Read the model definition and answer for the solid it produces. Units are mm, in the model's axes. A direction names the side the tool comes from. Give positions to 0.01 mm unless a question says otherwise; leave off trailing zeros. Loops run counter-clockwise (first coordinate to the right, second up) from the corner with the lowest first, then second, coordinate; pieces in that order, holes last.
(1) Find section C-C, the plane z = -3.25. Write down the section's boundary in (x, y), then the cut area to 3 significant figures.
(2) Each of these flat-tipped pins is pushed along its axis until it touches: P1, Ø2.5, axis at x = -12, y = 3, coming from the -Z side; P2, Ø1, axis at y = 0.5, z = 1, coming from the +X side; P3, Ø2, axis at x = -3, y = 3, coming from the -Z side. Where does it stop, or does it pass through?
(3) Straight lines are drawn through the part: probe 1 along X at (y, z) = (1.5, -1); probe 2 along X at (y, z) = (3.6, 3.75); probe 3 along Z at (x, y) = (-5, 4). For each, find the intervals that lie inside material, in ascending order.
(4) Determine the mould class of faces 4 (the face through (-11.463, 2.465, 3.063)), 5 (the face through (-2, 0, 1)), 6 (the face through (5.96, 2.46, 4.49)), 7 (the face through (-12, 2, 0)) for opening direction Z: pulls with the +Z half, pulls with the -Z half, needs draft (parallel to the pull), parting line crosses it, or undercut.
(5) Which of the six approach directions +Z, -Z, +X, -X, +Y, -Y give full straight-line access (tool end or side, diameter ignored) to faces 1 (the face through (-11.82, 2.46, 1.03)), 2 (the face through (-5.02, 2.46, 10.75)), 3 (the face through (0.593, 2.465, 7.521))?
(6) Find section D-D, the plane y = 4.2. State how many separate pieces and enclosed holes the cut face has, then the cut area to 3 significant figures.
(7) Find section B-B, the plane x = 7.5. Write down the section's boundary in (y, z).
(8) Find section A-A, the plane z = -0.75. Write down the section's boundary in (x, y), then the cut area to 3 significant figures.
```python
from build123d import *

# Parameters (mm, degrees)
ESQUISSE1_R        = 1
ESQUISSE1_R_2      = 1.5
BOSS_EXTRU_1_DEPTH = 5


with BuildPart() as part:
    # Esquisse1 → Boss.-Extru.1 (new body)
    with BuildSketch(Plane(origin=(0, 0, 0), x_dir=(1, 0, 0), z_dir=(0, 1, 0))):
        with BuildLine():
            Line((3.99317755, -3.009075116), (7.9863551, -6.018150232))
            ThreePointArc((7.9863551, -6.018150232), (3.173046564, 9.483236552), (-10, 0))
            Line((-10, 0), (-13.125, 0))
            ThreePointArc((-13.125, 0), (-13.034258246, -0.270986186), (-12.798628832, -0.432684541))
            Line((-12.798628832, -0.432684541), (-12.167425855, -0.613035071))
            ThreePointArc((-12.167425855, -0.613035071), (-11.81998128, -1.034114365), (-12.089027739, -1.509129635))
            Line((-12.089027739, -1.509129635), (-12.679323783, -1.796347483))
            ThreePointArc((-12.679323783, -1.796347483), (-12.925601758, -2.279132332), (-12.529054019, -2.648569664))
            Line((-12.529054019, -2.648569664), (-11.876122893, -2.716573018))
            ThreePointArc((-11.876122893, -2.716573018), (-11.46083713, -3.070922054), (-11.643310633, -3.585440202))
            Line((-11.643310633, -3.585440202), (-12.174763898, -3.970798397))
            ThreePointArc((-12.174763898, -3.970798397), (-12.333465648, -4.489014381), (-11.878790241, -4.783979338))
            Line((-11.878790241, -4.783979338), (-11.223969947, -4.737569268))
            ThreePointArc((-11.223969947, -4.737569268), (-10.753461244, -5.01442133), (-10.843817425, -5.552808982))
            Line((-10.843817425, -5.552808982), (-11.300279972, -6.024598612))
            ThreePointArc((-11.300279972, -6.024598612), (-11.366583425, -6.5625), (-10.867595431, -6.77403022))
            Line((-10.867595431, -6.77403022), (-10.230782353, -6.614616873))
            ThreePointArc((-10.230782353, -6.614616873), (-9.719346879, -6.805559951), (-9.714840312, -7.351458472))
            Line((-9.714840312, -7.351458472), (-10.082442758, -7.895344446))
            ThreePointArc((-10.082442758, -7.895344446), (-10.054333316, -8.436587377), (-9.526194234, -8.558255622))
            Line((-9.526194234, -8.558255622), (-8.926737615, -8.290682691))
            ThreePointArc((-8.926737615, -8.290682691), (-8.389915077, -8.389915077), (-8.290682691, -8.926737615))
            Line((-8.290682691, -8.926737615), (-8.558255622, -9.526194234))
            ThreePointArc((-8.558255622, -9.526194234), (-8.436587377, -10.054333316), (-7.895344446, -10.082442758))
            Line((-7.895344446, -10.082442758), (-7.351458472, -9.714840312))
            ThreePointArc((-7.351458472, -9.714840312), (-6.805559951, -9.719346879), (-6.614616873, -10.230782353))
            Line((-6.614616873, -10.230782353), (-6.77403022, -10.867595431))
            ThreePointArc((-6.77403022, -10.867595431), (-6.5625, -11.366583425), (-6.024598612, -11.300279972))
            Line((-6.024598612, -11.300279972), (-5.552808982, -10.843817425))
            ThreePointArc((-5.552808982, -10.843817425), (-5.01442133, -10.753461244), (-4.737569268, -11.223969947))
            Line((-4.737569268, -11.223969947), (-4.783979338, -11.878790241))
            ThreePointArc((-4.783979338, -11.878790241), (-4.489014381, -12.333465648), (-3.970798397, -12.174763898))
            Line((-3.970798397, -12.174763898), (-3.585440202, -11.643310633))
            ThreePointArc((-3.585440202, -11.643310633), (-3.070922054, -11.46083713), (-2.716573018, -11.876122893))
            Line((-2.716573018, -11.876122893), (-2.713178959, -11.908710794))
            Line((-2.713178959, -11.908710794), (3.99317755, -3.009075116))
        make_face()
        with Locations(Location((-4.814520185, -6.38908408, 0), (0, 0, 270))):
            Circle(ESQUISSE1_R, mode=Mode.SUBTRACT)
        with Locations(Location((0, 0, 0), (0, 0, 270))):
            Circle(ESQUISSE1_R_2, mode=Mode.SUBTRACT)
    extrude(amount=BOSS_EXTRU_1_DEPTH)


solid = part.part
```
Entries:
1. outline: (-9.46, 0) - (9.46, 0) - (9.46, 5) - (-9.46, 5) - close
1. area: 94.6 mm2
2. P1: stops at z = 0
2. P2: stops at x = 9.99
2. P3: stops at z = -9.8
3. probe 1: x = -9.95 to -1.12, 1.12 to 9.95
3. probe 2: x = -11.87 to 3.43, 4.98 to 9.27
3. probe 3: z = -8.66 to 5.41, 7.37 to 10.76
4. face 4: undercut
4. face 5: needs draft
4. face 6: pulls with the +Z half
4. face 7: pulls with the -Z half
5. face 1: -X, +Y, -Y
5. face 2: +Y, -Y
5. face 3: +Z, +Y, -Y
6. separate pieces: 1
6. enclosed holes: 2
6. area: 312 mm2
7. outline: (0, -6.61) - (5, -6.61) - (5, 5.65) - (0, 5.65) - close
8. outline: (-9.97, 0) - (-1.3, 0) - (-1.3, 5) - (-9.97, 5) - close; (1.3, 0) - (9.97, 0) - (9.97, 5) - (1.3, 5) - close
8. area: 86.7 mm2
